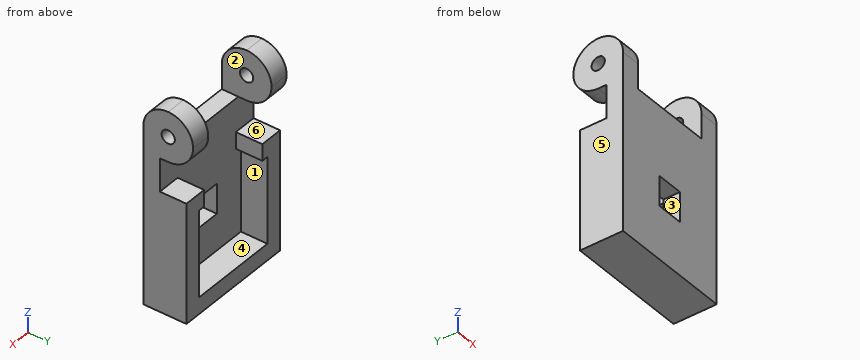
```python
from build123d import *

# Parameters (mm, degrees)
SKIZZE1_W                            = 37
SKIZZE1_H                            = 46
SKIZZE1_W_2                          = 25
SKIZZE1_H_2                          = 24
SKIZZE1_W_3                          = 8
SKIZZE1_H_3                          = 9
AUFSATZ_LINEAR_AUSTRAGEN2_DEPTH      = 5
AUFSATZ_LINEAR_AUSTRAGEN3_DEPTH      = 8
AUFSATZ_LINEAR_AUSTRAGEN4_DEPTH      = 37
SCHNITT_LINEAR_AUSTRAGEN1_DEPTH      = 22
SCHNITT_LINEAR_AUSTRAGEN1_DEPTH_BACK = 11
SKIZZE4_W                            = 25
SKIZZE4_H                            = 15


with BuildPart() as part:
    # Skizze1 → Aufsatz-Linear austragen2 (new body)
    # profile 1 of 2: a face of its own
    with BuildSketch(Plane(origin=(0, 0, 0), x_dir=(1, 0, 0), z_dir=(0, 1, 0))):
        with Locations((0, -2.5)):
            Rectangle(SKIZZE1_W, SKIZZE1_H)
        with Locations((0, 2.5)):
            Rectangle(SKIZZE1_W_2, SKIZZE1_H_2, mode=Mode.SUBTRACT)
    # profile 2 of 2: a face of its own
    with BuildSketch(Plane(origin=(0, 0, 0), x_dir=(1, 0, 0), z_dir=(0, 1, 0))):
        with Locations((0, 2.5)):
            Rectangle(SKIZZE1_W_2, SKIZZE1_H_2)
        Rectangle(SKIZZE1_W_3, SKIZZE1_H_3, mode=Mode.SUBTRACT)
    extrude(amount=AUFSATZ_LINEAR_AUSTRAGEN2_DEPTH)

    # Skizze2 → Aufsatz-Linear austragen3 (add)
    with BuildSketch(Plane(origin=(0, 5, 0), x_dir=(1, 0, 0), z_dir=(0, 1, 0))):
        Polygon((-13.5, -10.5), (-13.5, 15.5), (13.5, 15.5), (13.5, -10.5), (18.5, -10.5), (18.5, 20.5), (-18.5, 20.5), (-18.5, -10.5), align=None)
        Polygon((-11.5, -10.5), (-13.5, -10.5), (-18.5, -10.5), (-18.5, -15.5), (-11.5, -15.5), align=None)
        Polygon((18.5, -10.5), (13.5, -10.5), (11.5, -10.5), (11.5, -15.5), (18.5, -15.5), align=None)
    extrude(amount=AUFSATZ_LINEAR_AUSTRAGEN3_DEPTH)

    # Skizze3 → Aufsatz-Linear austragen4 (add)
    with BuildSketch(Plane.ZY.offset(18.5)):
        with BuildLine():
            Line((25.5, 0), (33, 0))
            ThreePointArc((33, 0), (27.696699141, 2.196699141), (25.5, 7.5))
            Line((25.5, 7.5), (25.5, 5))
            Line((25.5, 5), (25.5, 0))
        make_face()
        with BuildLine():
            ThreePointArc((31, 7.5), (33, 9.5), (35, 7.5))
            Line((35, 7.5), (40.5, 7.5))
            ThreePointArc((40.5, 7.5), (38.303300859, 12.803300859), (33, 15))
            ThreePointArc((33, 15), (27.696699141, 12.803300859), (25.5, 7.5))
            Line((25.5, 7.5), (31, 7.5))
        make_face()
        with BuildLine():
            Line((40.5, 7.5), (35, 7.5))
            ThreePointArc((35, 7.5), (33, 5.5), (31, 7.5))
            Line((31, 7.5), (25.5, 7.5))
            ThreePointArc((25.5, 7.5), (27.696699141, 2.196699141), (33, 0))
            ThreePointArc((33, 0), (38.303300859, 2.196699141), (40.5, 7.5))
        make_face()
    extrude(amount=-AUFSATZ_LINEAR_AUSTRAGEN4_DEPTH)

    # Skizze4 → Schnitt-Linear austragen1 (cut, two sides: drawn at the far end of the back side and taken through both)
    with BuildSketch(Plane(origin=(0, 5, 0), x_dir=(1, 0, 0), z_dir=(0, 1, 0)).offset(-SCHNITT_LINEAR_AUSTRAGEN1_DEPTH_BACK)):
        with Locations((0, -33)):
            Rectangle(SKIZZE4_W, SKIZZE4_H)
    extrude(amount=SCHNITT_LINEAR_AUSTRAGEN1_DEPTH + SCHNITT_LINEAR_AUSTRAGEN1_DEPTH_BACK, mode=Mode.SUBTRACT)


solid = part.part
```
Geometry check sheet. Reference: the model listing, model coordinates, mm. Face numbers are marked on the shaded views. A direction names the side the tool comes from. Round coordinates to 2 decimals unless told otherwise and drop trailing zeros. Loops run counter-clockwise (first coordinate to the right, second up) from the corner with the lowest first, then second, coordinate; pieces in that order, holes last. Notation, with made-up numbers: (59, 33) - (73, 33) arc R15 ccw to (73, 51) - close; hole circle Ø3 at (5, 21.25). An arc over 180 degrees is marked (long way). Write item = value, one per line. Start each with the question number.
1. Set-up check for the marked faces 1, 2 and 3: record each of +Z, -Z, +X, -X, +Y, -Y from which the full face is reachable in a straight line by a thin tool's end or side.
2. Section check B-B on y = 3. Enter the section's corners in (x, z).
3. Section check D-D on x = 15.5. Enter the section's corners in (y, z), then the cut area to 3 significant figures.
4. Thickness scan on line 1 (Z direction, x = 14.3, y = 7.5); line 2 (X direction, y = 10.75, z = -14.5); line 3 (Z direction, x = -16, y = 7). Record the ranges inside material, lowest first.
5. Section check A-A on z = 1. Enter the section's corners in (x, y), then the cut area to 3 significant figures.
6. Mould release check, pull along X, two halves, no side actions. Record for the marked faces 4, 5 and 6: released by +X, released by -X, zero draft, split by the parting line, or undercut.
7. Section check C-C on x = -0.5. Enter the section's corners in (y, z), then the cut area to 3 significant figures.
8. Depth check by flat-ended pin: pin 1 (4 mm diameter, centred on x = -10, y = 9, fed in from +Z); pin 2 (5.5 mm diameter, centred on x = 3, y = 3.5, fed in from +Z). Enter the tip coordinate at first touch or a pass-through.
Working result:
q1.face_1 = +Y
q1.face_2 = +Z, +Y, -Y
q1.face_3 = +Y, -Y
q2.outline = (-18.5, -20.5) - (18.5, -20.5) - (18.5, 39) - (12.5, 39) - (12.5, 25.5) - (-12.5, 25.5) - (-12.5, 39) - (-18.5, 39) - close; hole (-4, -4.5) - (4, -4.5) - (4, 4.5) - (-4, 4.5) - close
q3.outline = (0, -20.5) - (13, -20.5) - (13, 15.5) - (5, 15.5) - (5, 25.5) - (7.5, 25.5) arc R7.5 ccw (long way) to (0, 33) - close; hole circle Ø4 at (7.5, 33)
q3.area = 694 mm^2
q4.line_1 = -20.5 to 15.5, 25.5 to 31, 35 to 40.5
q4.line_2 = -18.5 to -13.5, 13.5 to 18.5
q4.line_3 = -20.5 to 15.5, 25.5 to 31.06, 34.94 to 40.48
q5.outline = (-18.5, 0) - (-4, 0) - (-4, 5) - (-13.5, 5) - (-13.5, 13) - (-18.5, 13) - close; (4, 0) - (18.5, 0) - (18.5, 13) - (13.5, 13) - (13.5, 5) - (4, 5) - close
q5.area = 225 mm^2
q6.face_4 = undercut
q6.face_5 = released by -X
q6.face_6 = zero draft
q7.outline = (0, -20.5) - (13, -20.5) - (13, -15.5) - (5, -15.5) - (5, -4.5) - (0, -4.5) - close; (0, 4.5) - (5, 4.5) - (5, 25.5) - (0, 25.5) - close
q7.area = 225 mm^2
q8.pin_1 = 15.5
q8.pin_2 = 25.5
